Could you check a few things on this model? Use its own coordinates, in mm. Face numbers are marked on the shaded views. Give positions to 0.01 mm unless a question says otherwise; leave off trailing zeros. Loops run counter-clockwise (first coordinate to the right, second up) from the corner with the lowest first, then second, coordinate; pieces in that order, holes last. Notation, with made-up numbers: (28.25, 86) -> (77.25, 86) arc R21 cw to (77.25, 96) -> close; hole circle Ø4 at (10.25, 81). An arc over 180 degrees is marked (long way). Put each result on its own line as item: value.
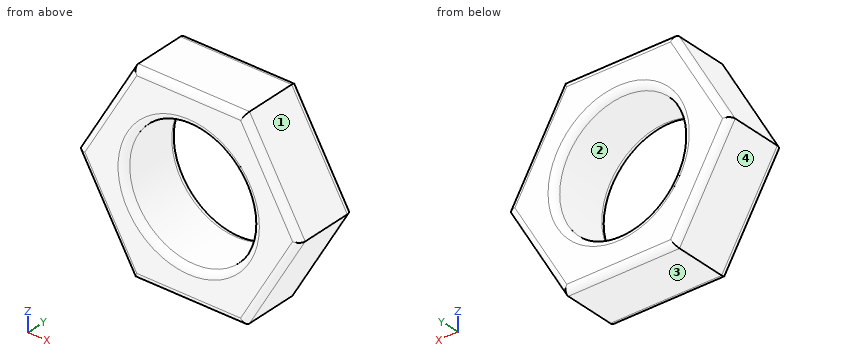
```python
from build123d import *

# Parameters (mm, degrees)
SKETCH1_R           = 5
BOSS_EXTRUDE1_DEPTH = 5
FILLET1_R           = 0.5


with BuildPart() as part:
    # Sketch1 → Boss-Extrude1 (new body)
    with BuildSketch(Plane(origin=(0, 0, 0), x_dir=(1, 0, 0), z_dir=(0, 1, 0))):
        Polygon((4.330127019, -7.5), (8.660254038, 0), (4.330127019, 7.5), (-4.330127019, 7.5), (-8.660254038, 0), (-4.330127019, -7.5), align=None)
        Circle(SKETCH1_R, mode=Mode.SUBTRACT)
    extrude(amount=BOSS_EXTRUDE1_DEPTH)

    # Fillet1
    fillet1_edges = [part.edges().sort_by_distance(p)[0] for p in [
        (6.495190528, 5, -3.75),
        (0, 5, -7.5),
        (-6.495190528, 5, -3.75),
        (-5, 0, 0),
        (-5, 5, 0),
        (-6.495190528, 5, 3.75),
        (0, 5, 7.5),
        (-6.495190528, 0, 3.75),
        (-6.495190528, 0, -3.75),
        (0, 0, -7.5),
        (6.495190528, 5, 3.75),
        (6.495190528, 0, -3.75),
        (6.495190528, 0, 3.75),
        (0, 0, 7.5),
    ]]
    fillet(fillet1_edges, radius=FILLET1_R)


solid = part.part
```
1. If we section it at A-A (x = 0): List the corners of the cut face in (y, z) for me.
Recorded:
outline: (0, -7) arc R0.5 ccw to (0.5, -7.5) -> (4.5, -7.5) arc R0.5 ccw to (5, -7) -> (5, -5.5) arc R0.5 ccw to (4.5, -5) -> (0.5, -5) arc R0.5 ccw to (0, -5.5) -> close; (0, 5.5) arc R0.5 ccw to (0.5, 5) -> (4.5, 5) arc R0.5 ccw to (5, 5.5) -> (5, 7) arc R0.5 ccw to (4.5, 7.5) -> (0.5, 7.5) arc R0.5 ccw to (0, 7) -> close
2. If we section it at B-B (y = 4.15): List the corners of the cut face in (x, z) for me, then the cut area to 3 significant figures.
Recorded:
outline: (-8.66, 0) -> (-4.33, -7.5) -> (4.33, -7.5) -> (8.66, 0) -> (4.33, 7.5) -> (-4.33, 7.5) -> close; hole circle Ø10 at (0, 0)
area: 116 mm^2
3. Thinking about a two-plate mould opening in X: for the marked faces 1, 2, 3 and 4, which applies, pulls with the +X half, pulls with the -X half, needs draft (parallel to the pull), parting line crosses it, or undercut?
Recorded:
face 1: pulls with the +X half
face 2: undercut
face 3: needs draft
face 4: pulls with the -X half
4. I need wall thicknesses on line 1 (Z direction, x = 0, y = 2.55); line 2 (X direction, y = 0.4, z = 0.75); line 3 (X direction, y = 3.85, z = 0.5). Which ranges of each line are inside material? Lowest first, please.
Recorded:
line 1: z = -7.5 to -5, 5 to 7.5
line 2: x = -8.22 to -4.95, 4.95 to 8.22
line 3: x = -8.37 to -4.97, 4.97 to 8.37
5. I'm going to push flat-ended pins straight in: pin 1 (2 mm diameter, centred on x = 6, y = 1, fed in from -Z); pin 2 (2 mm diameter, centred on y = 1, z = -5.5, fed in from -X); pin 3 (2 mm diameter, centred on y = 1, z = -3.5, fed in from -X). Where does each tip first touch, or does it pass through?
Recorded:
pin 1: stops at z = -6.34
pin 2: stops at x = -6.06
pin 3: stops at x = -7.22
